Part model, mm, in its own coordinate system. A direction names the side the tool comes from. Round coordinates to 2 decimals unless told otherwise and drop trailing zeros. Loops run counter-clockwise (first coordinate to the right, second up) from the corner with the lowest first, then second, coordinate; pieces in that order, holes last. Notation, with made-up numbers: (-10.75, -19) -> (5.25, -19) arc R20 ccw to (5.25, -14) -> close; hole circle Ø3 at (88, 39.25). An arc over 180 degrees is marked (long way). Answer as CSV lines item,"result".
from build123d import *

# Parameters (mm, degrees)
ESQUISSE1_R             = 3
ESQUISSE1_R_2           = 2.5
ESQUISSE1_W             = 40
ESQUISSE1_H             = 8
BOSS_EXTRU_1_DEPTH      = 6
ESQUISSE2_R             = 2.5
BOSS_EXTRU_2_DEPTH      = 8
CONG_2_R                = 2
ENL_V_MAT_EXTRU_1_DEPTH = 4
ENL_V_START             = -10
ENL_V_MAT_EXTRU_4_DEPTH = 10


with BuildPart() as part:
    # Esquisse1 → Boss.-Extru.1 (new body)
    with BuildSketch(Plane.XY):
        with BuildLine():
            Line((90, -15), (-90, -15))
            ThreePointArc((-90, -15), (-105, 0), (-90, 15))
            Line((-90, 15), (90, 15))
            ThreePointArc((90, 15), (105, 0), (90, -15))
        make_face()
        with Locations((90, 0)):
            Circle(ESQUISSE1_R, mode=Mode.SUBTRACT)
        with Locations(Location((-90, 0, 0), (0, 0, 180))):
            Circle(ESQUISSE1_R, mode=Mode.SUBTRACT)
        Circle(ESQUISSE1_R_2, mode=Mode.SUBTRACT)
        with Locations((-57.5, 0)):
            Circle(ESQUISSE1_R_2, mode=Mode.SUBTRACT)
        with Locations((-30, 0)):
            Circle(ESQUISSE1_R_2, mode=Mode.SUBTRACT)
        with Locations((60, 0)):
            Rectangle(ESQUISSE1_W, ESQUISSE1_H, mode=Mode.SUBTRACT)
    extrude(amount=BOSS_EXTRU_1_DEPTH)

    # Esquisse2 → Boss.-Extru.2 (add)
    with BuildSketch(Plane(origin=(40, 0, 0), x_dir=(0, 0, -1), z_dir=(1, 0, 0))):
        Polygon((-16, 5), (-16, -5), (-6, -15), (-6, -5), (-6, 5), (-6, 15), align=None)
        with Locations((-11, 0)):
            Circle(ESQUISSE2_R, mode=Mode.SUBTRACT)
    extrude(amount=-BOSS_EXTRU_2_DEPTH)

    # Congé2
    cong_2_edges = [part.edges().sort_by_distance(p)[0] for p in [
        (40, 9.5, 6),
        (40, -9.5, 6),
    ]]
    fillet(cong_2_edges, radius=CONG_2_R)

    # Esquisse3 → Enlèv. mat.-Extru.1 (cut)
    with BuildSketch(Plane.ZY.offset(-32)):
        Polygon((11, 4), (14.464101615, 2), (14.464101615, -2), (11, -4), (7.535898385, -2), (7.535898385, 2), align=None)
    extrude(amount=-ENL_V_MAT_EXTRU_1_DEPTH, mode=Mode.SUBTRACT)

    # Esquisse4 → Enlèv. mat.-Extru.4 (cut)
    with BuildSketch(Plane.XY.offset(6).offset(ENL_V_START)):
        with BuildLine():
            ThreePointArc((-105, 0), (-104.771638598, -1.148050297), (-104.121320344, -2.121320344))
            Line((-104.121320344, -2.121320344), (-99.878679656, 2.121320344))
            ThreePointArc((-99.878679656, 2.121320344), (-103.148050297, 2.771638598), (-105, 0))
        make_face()
        with BuildLine():
            Line((-99.878679656, 2.121320344), (-104.121320344, -2.121320344))
            ThreePointArc((-104.121320344, -2.121320344), (-100.851949703, -2.771638598), (-99, 0))
            ThreePointArc((-99, 0), (-99.228361402, 1.148050297), (-99.878679656, 2.121320344))
        make_face()
        with BuildLine():
            ThreePointArc((-105, 0), (-103.148050297, 2.771638598), (-99.878679656, 2.121320344))
            Line((-99.878679656, 2.121320344), (-103.750652313, 5.993293))
            ThreePointArc((-103.750652313, 5.993293), (-104.68434174, 3.061063158), (-105, 0))
        make_face()
        with BuildLine():
            Line((-104.94364809, -1.298992597), (-104.121320344, -2.121320344))
            ThreePointArc((-104.121320344, -2.121320344), (-104.771638598, -1.148050297), (-105, 0))
            ThreePointArc((-105, 0), (-104.985905401, -0.650107165), (-104.94364809, -1.298992597))
        make_face()
        with BuildLine():
            ThreePointArc((-105, 0), (-104.771638598, -1.148050297), (-104.121320344, -2.121320344))
            Line((-104.121320344, -2.121320344), (-99.878679656, 2.121320344))
            ThreePointArc((-99.878679656, 2.121320344), (-103.148050297, 2.771638598), (-105, 0))
        make_face()
        with BuildLine():
            Line((-99.878679656, 2.121320344), (-104.121320344, -2.121320344))
            ThreePointArc((-104.121320344, -2.121320344), (-100.851949703, -2.771638598), (-99, 0))
            ThreePointArc((-99, 0), (-99.228361402, 1.148050297), (-99.878679656, 2.121320344))
        make_face()
    extrude(amount=ENL_V_MAT_EXTRU_4_DEPTH, mode=Mode.SUBTRACT)


solid = part.part
Q1. Which spindle directions (+Z, -Z, +X, -X, +Y, -Y) get a long thin tool onto all of the face, cutting with end or side? Do faces 4 (the face through (1, -15, 3)), 5 (the face through (-101.79, 4.03, 2.96)), 6 (the face through (33.972, 2.986, 9.244)), 7 (the face through (-36, 0, 6)), 8 (the face through (60, 4, 3)). Say none if no direction does.
Geometry results:
face 4,"+Z, -Z, +X, -X, -Y"
face 5,"+Z, -Z, -X"
face 6,"-X"
face 7,"+Z, -X, +Y, -Y"
face 8,"+Z, -Z"
Q2. Saw through at D-D, the plane y = 8. Write the cut outline in (x, z), then the cut area to 3 significant figures.
Geometry results:
outline,"(-102.69, 0) -> (102.69, 0) -> (102.69, 6) -> (42, 6) arc R2 cw to (40, 8) -> (40, 13) -> (32, 13) -> (32, 6) -> (-102.69, 6) -> close"
area,"1,290 mm2"
Q3. Saw through at B-B, the plane z = 3. Write the cut outline in (x, y), then the cut area to 3 significant figures.
Geometry results:
outline,"(-104.94, -1.3) arc R15 ccw to (-90, -15) -> (90, -15) arc R15 ccw to (90, 15) -> (-90, 15) arc R15 ccw to (-103.75, 5.99) -> (-99.88, 2.12) arc R3 cw to (-104.12, -2.12) -> close; hole circle Ø6 at (-90, 0); hole circle Ø5 at (-57.5, 0); hole circle Ø5 at (-30, 0); hole circle Ø5 at (0, 0); hole (40, -4) -> (80, -4) -> (80, 4) -> (40, 4) -> close; hole circle Ø6 at (90, 0)"
area,"5,640 mm2"
Q4. Saw through at A-A, the plane x = -30. Write the cut outline in (y, z).
Geometry results:
outline,"(-15, 0) -> (-2.5, 0) -> (-2.5, 6) -> (-15, 6) -> close; (2.5, 0) -> (15, 0) -> (15, 6) -> (2.5, 6) -> close"
Q5. Two-plate mould, pull along Z, no slides. Class faces 1 (the face through (36, 10, 11)), 2 (the face through (105, 0, 3)), 3 (the face through (33.972, -2.986, 12.756)): pulls with the +Z half, pulls with the -Z half, needs draft (parallel to the pull), parting line crosses it, or undercut.
Geometry results:
face 1,"pulls with the +Z half"
face 2,"needs draft"
face 3,"undercut"
Q6. Drill centre lines: line 1 along Y through (x, z) = (0, 3.5); line 2 along Y through (x, z) = (90, 3.35); line 3 along Z through (x, y) = (74.5, -7). Where is each one in solid material? Low to high.
Geometry results:
line 1,"-15 to -2.5, 2.5 to 15"
line 2,"-15 to -3, 3 to 15"
line 3,"0 to 6"
Q7. Saw through at C-C, the plane x = 58. Write the cut outline in (y, z), then the cut area to 3 significant figures.
Geometry results:
outline,"(-15, 0) -> (-4, 0) -> (-4, 6) -> (-15, 6) -> close; (4, 0) -> (15, 0) -> (15, 6) -> (4, 6) -> close"
area,"132 mm2"
Q8. Drop flat-ended pins along their axis: P1, Ø1.5, axis at x = -64, y = 10.5, coming from the -Z side; P2, Ø5.5, axis at y = -0.5, z = 9.5, coming from the -X side; P3, Ø4, axis at x = -80, y = 8.5, coming from the +Z side. Give the stop position or say it passes through.
Geometry results:
P1,"z = 0"
P2,"x = 32"
P3,"z = 6"
